```python
from build123d import *

# Parameters (mm, degrees)
F1_DEPTH       = 204
F5_DEPTH       = 2
F7_D           = 5
F7_DEPTH       = 10
F7_CSINK_D     = 8
F7_CSINK_ANGLE = 90
F8_D           = 5
F8_DEPTH       = 10
F8_CSINK_D     = 8
F8_CSINK_ANGLE = 90


with BuildPart() as f1:
    # F0 (on Front) → F1 (new body)
    with BuildSketch(Plane.XZ):
        Polygon((30, 0), (30, 31.041134), (-371.513106, 312.183638), (-375, 312.183638), (28, 30), (28, 0), align=None)
    extrude(amount=F1_DEPTH)

    # F4 (on offset) → F5 (join)
    with BuildSketch(Plane.XZ.offset(204)):
        Polygon((0, 52.04736), (0, 0), (30, 0), (30, 31.041134), align=None)
        Polygon((-265, 237.602358), (-315, 272.612735), (-315, 242.612735), (-265, 207.602358), align=None)
    extrude(amount=F5_DEPTH)

    # F7
    with Locations(Plane.XZ.offset(206)):
        with Locations((15, 23.274141), (15, 9.274141)):
            CounterSinkHole(F7_D / 2, F7_CSINK_D / 2, depth=F7_DEPTH, counter_sink_angle=F7_CSINK_ANGLE)

    # F8
    with Locations(Plane.XZ.offset(206)):
        with Locations((-305, 247.299041), (-275, 226.292814)):
            CounterSinkHole(F8_D / 2, F8_CSINK_D / 2, depth=F8_DEPTH, counter_sink_angle=F8_CSINK_ANGLE)

    # F9: F1 across plane


with BuildPart() as f1_1:
    add(f1.part)
    add(f1.part.mirror(Plane.XZ.offset(102)))


solid = f1_1.part
```
Here's how the part is built. I have some questions about the finished solid (model axes, mm). A direction names the side the tool comes from. Coordinates: 2 decimals unless noted, no trailing zeros. Order: outer loops, then holes, each group sorted by start corner. A loop starts at its lowest first (then second) coordinate and runs counter-clockwise, first axis right, second up.
Item 1: Thinking about a two-plate mould opening in Y: for faces 3 (the face through (-133, 0, 144)), 4 (the face through (-290, 0, 239)), 5 (the face through (-290.35, 0.986, 225.353)), which applies, pulls with the +Y half, pulls with the -Y half, needs draft (parallel to the pull), parting line crosses it, or undercut?
Response values:
face 3: pulls with the +Y half
face 4: undercut
face 5: needs draft
Item 2: If we section it at B-B, the plane x = -214.5: List the corners of the cut face in (y, z) for me.
Response values:
outline: (-204, 199.8) - (0, 199.8) - (0, 202.24) - (-204, 202.24) - close
Item 3: If we section it at A-A, the plane y = -69.5: List the corners of the cut face in (x, z) for me, then the cut area to 3 significant figures.
Response values:
outline: (-375, 312.18) - (28, 30) - (28, 0) - (30, 0) - (30, 31.04) - (-371.51, 312.18) - close
area: 1,040 mm2
Item 4: I need wall thicknesses on probe 1 along Z at (x, y) = (15, 0.35); probe 2 along Z at (x, y) = (-275, -204.25); probe 3 along X at (y, z) = (-120.5, 27). Which ranges of each line are inside material? Lowest first, please.
Response values:
probe 1: z = 0 to 6.77, 11.77 to 20.77, 25.77 to 41.54
probe 2: z = 214.6 to 223.79, 228.79 to 244.6
probe 3: x = 28 to 30
Item 5: Which directions (+Z, -Z, +X, -X, +Y, -Y) give clear straight access to the entire face, cutting with the end or side of a thin tool? Please do faces 1 (the face through (28, -101, 15)), 2 (the face through (-290.35, -204.986, 225.353)).
Response values:
face 1: -Z, -X
face 2: -Z, -X, +Y, -Y
Item 6: I'm going to push flat-ended pins straight in: pin 1 Ø2 at (y, z) = (0.5, 217.5) entering from +X; pin 2 Ø5 at (y, z) = (-20, 43) entering from +X; pin 3 Ø1 at (y, z) = (-205, 28) entering from -X. Where does each tip first touch, or does it pass through?
Response values:
pin 1: stops at x = -235.05
pin 2: stops at x = 16.49
pin 3: stops at x = 0
